Could you check a few things on this model? Use its own coordinates, in mm. A direction names the side the tool comes from. Round coordinates to 2 decimals unless told otherwise and drop trailing zeros. Order: outer loops, then holes, each group sorted by start corner. A loop starts at its lowest first (then second) coordinate and runs counter-clockwise, first axis right, second up. Notation, with made-up numbers: M 87.25,-33 L 128.25,-33 A10 ccw 128.25,-25 Z; hole C 22.25,-28.5 d4. An arc over 180 degrees is marked long. Write each question's results on one line, items separated by ' | '. Start each with the question number.
1. Suppose I cut it at A-A on z = 0. Write out the boundary of the cut face in (x, y).
2. I'm going to push flat-ended pins straight in: pin 1 (4 mm diameter, centred on y = 11, z = -7, fed in from -X); pin 2 (8 mm diameter, centred on x = 7.18, z = 0, fed in from +Y); pin 3 (1.5 mm diameter, centred on x = 0.5, z = 1, fed in from +Y); pin 4 (3 mm diameter, centred on y = 14, z = 0, fed in from +X). Where does each tip first touch, or does it pass through?
3. Suppose I cut it at B-B on x = -1.5. Write out the boundary of the cut face in (y, z), and give its area (3 significant figures).
4. We'd pull the mould along Z, two halves only. Please class faces 5 (the flat face through (-15.764, 14, 0)), 6 (the cylindrical face through (-6.6, 14.4, -9.5)), 7 (the flat face through (-7, 5, 0)): released by +Z, released by -Z, zero draft, split by the parting line, or undercut.
5. Suppose I cut it at C-C on z = 7. Write out the boundary of the cut face in (x, y), and give its area (3 significant figures).
6. For faces 1 (the cylindrical face through (-6.96, 14.39, 9.5)), 2 (the flat face through (2.18, 14, 0)), 3 (the flat face through (-25.842, 2, 0)), 4 (the flat face through (-11, 5, -9)), which set-ups out of +Z, -Z, +X, -X, +Y, -Y let a thin tool reach every point of the face, with its end or its side?
7. Suppose I cut it at D-D on x = 8. Write out the boundary of the cut face in (y, z), and give its area (3 significant figures).
8. Please list where these lines run through material, in increasing order: L1, parallel to X at y = 2.05, z = 0; L2, parallel to X at y = 17.25, z = 0; L3, parallel to Y at x = 4, z = 3.75.
from build123d import *

# Parameters (mm, degrees)
SKETCH1_W           = 38.1
SKETCH1_H           = 25.4
BOSS_EXTRUDE1_DEPTH = 5
SKETCH3_R           = 9.5
SKETCH3_R_2         = 7.75
BOSS_EXTRUDE2_DEPTH = 19.05
SKETCH4_R           = 3.5
CUT_EXTRUDE1_DEPTH  = 35.525178946
SKETCH5_W           = 1.6
SKETCH5_H           = 10
CUT_EXTRUDE2_DEPTH  = 35.525178946


with BuildPart() as part:
    # Sketch1 → Boss-Extrude1 (new body)
    with BuildSketch(Plane(origin=(0, 0, 0), x_dir=(1, 0, 0), z_dir=(0, 1, 0))):
        with Locations((-6.79173913, 0)):
            Rectangle(SKETCH1_W, SKETCH1_H)
    extrude(amount=BOSS_EXTRUDE1_DEPTH)

    # Sketch3 → Boss-Extrude2 (add)
    with BuildSketch(Plane(origin=(0, 5, 0), x_dir=(1, 0, 0), z_dir=(0, 1, 0))):
        with Locations(Location((-6.79173913, 0, 0), (0, 0, 90))):
            Circle(SKETCH3_R)
        with Locations(Location((-6.79173913, 0, 0), (0, 0, 90))):
            Circle(SKETCH3_R_2, mode=Mode.SUBTRACT)
    extrude(amount=BOSS_EXTRUDE2_DEPTH)

    # Sketch4 → Cut-Extrude1 (cut, through all)
    with BuildSketch(Plane(origin=(0, 5, 0), x_dir=(1, 0, 0), z_dir=(0, 1, 0))):
        with Locations(Location((7.17826087, 0, 0), (0, 0, 270))):
            Circle(SKETCH4_R)
        with Locations(Location((-20.76173913, 0, 0), (0, 0, 270))):
            Circle(SKETCH4_R)
    extrude(amount=-CUT_EXTRUDE1_DEPTH, mode=Mode.SUBTRACT)

    # Sketch5 → Cut-Extrude2 (cut, through all)
    with BuildSketch(Plane(origin=(0, 5, 0), x_dir=(1, 0, 0), z_dir=(0, 1, 0))):
        with Locations((-16.563639087, -0.415081282)):
            Rectangle(SKETCH5_W, SKETCH5_H)
        with Locations((2.980160826, -0.415081282)):
            Rectangle(SKETCH5_W, SKETCH5_H)
    extrude(amount=CUT_EXTRUDE2_DEPTH, mode=Mode.SUBTRACT)


solid = part.part
Filled sheet:
1) outline: M -25.84,0 L -24.26,0 L -24.26,5 L -25.84,5 Z; M -17.26,0 L 3.68,0 L 3.68,5 L 2.18,5 L 2.18,24.05 L 0.96,24.05 L 0.96,5 L -14.54,5 L -14.54,24.05 L -15.76,24.05 L -15.76,5 L -17.26,5 Z; M 10.68,0 L 12.26,0 L 12.26,5 L 10.68,5 Z
2) pin 1: stops at x = -14.87 | pin 2: stops at y = 5 | pin 3: stops at y = 24.05 | pin 4: stops at x = 2.18
3) outline: M 0,-12.7 L 5,-12.7 L 5,-7.89 L 24.05,-7.89 L 24.05,-5.66 L 5,-5.66 L 5,5.66 L 24.05,5.66 L 24.05,7.89 L 5,7.89 L 5,12.7 L 0,12.7 Z | area: 212 mm^2
4) face 5: zero draft | face 6: released by -Z | face 7: undercut
5) outline: M -25.84,0 L 12.26,0 L 12.26,5 L -0.37,5 L -0.37,24.05 L -3.47,24.05 L -3.47,5 L -10.12,5 L -10.12,24.05 L -13.21,24.05 L -13.21,5 L -25.84,5 Z | area: 308 mm^2
6) face 1: +Z, +Y | face 2: +Z, -Z, +X, +Y | face 3: +Z, -Z, -X, +Y, -Y | face 4: +Y
7) outline: M 0,-12.7 L 5,-12.7 L 5,-3.4 L 0,-3.4 Z; M 0,3.4 L 5,3.4 L 5,12.7 L 0,12.7 Z | area: 93.0 mm^2
8) L1: x = -25.84 to -24.26, -17.26 to 3.68, 10.68 to 12.26 | L2: x = -15.76 to -14.54, 0.96 to 2.18 | L3: y = 0 to 5
